Autodesk Inventor part; units mm, degrees
ref_plane "YZ Plane" through (0, 0, 0) normal (1, 0, 0) x (0, 1, 0)
ref_plane "XZ Plane" through (0, 0, 0) normal (0, 1, 0) x (-1, 0, 0)
ref_plane "XY Plane" through (0, 0, 0) normal (0, 0, 1) x (1, 0, 0)
sketch "Sketch7" plane through (0, 0, 0) normal (0, 0, 1) x (1, 0, 0)
  line L0 (125, -75) -> (-125, -75)
  line L1 (-125, -75) -> (-125, 75)
  line L2 (-125, 75) -> (125, 75)
  line L3 (125, 75) -> (125, -75)
  line L4 (125, -75) -> (-125, 75) construction
  line L5 (-125, -75) -> (125, 75) construction
  point P0 (0, 0)
  dimension "d15" = 250
  dimension "d16" = 150
extrude "Box Outside" add sketch "Sketch7" along normal blind 60
sketch "Sketch8" plane through (0, 0, 60) normal (0, 0, 1) x (1, 0, 0)
  line L0 (-122, 72) -> (122, 72)
  line L1 (122, 72) -> (122, -72)
  line L2 (122, -72) -> (-122, -72)
  line L3 (-122, -72) -> (-122, 72)
  line L4 (125, 75) -> (-125, 75)
  line L5 (-125, 75) -> (-125, -75)
  line L6 (-125, -75) -> (125, -75)
  line L7 (125, -75) -> (125, 75)
  point P0 (0, 0)
  dimension "d19" = 3
  dimension "d20" = 3
  dimension "d21" = 3
  dimension "d22" = 3
extrude "Box Cut" cut sketch "Sketch8" against normal blind 55 contours L0 L1 L2 L3
sketch "Sketch9" plane through (-122, -72, 60) normal (0, 1, 0) x (1, 0, 0)
  line L0 (0, 0) -> (10, 0)
  line L1 (10, 0) -> (10, 25)
  line L2 (10, 25) -> (0, 25)
  line L3 (0, 25) -> (0, 0)
  point P0 (122, 60)
  dimension "d25" = 10
  dimension "d26" = 25
extrude "ScrewHole Box LB" add sketch "Sketch9" along normal blind 15
sketch "Sketch10" plane through (-122, -72, 5) normal (0, 1, 0) x (1, 0, 0)
  line L0 (244, -55) -> (244, 0)
  line L1 (244, -55) -> (234, -55)
  line L2 (234, -55) -> (234, -30)
  line L3 (234, -30) -> (244, -30)
  line L4 (244, -30) -> (244, -55)
  point P0 (122, 5)
  dimension "d29" = 10
  dimension "d30" = 25
extrude "ScrewHole Box RB" add sketch "Sketch10" along normal blind 15
sketch "Sketch11" plane through (-122, 72, 60) normal (0, -1, 0) x (1, 0, 0)
  line L0 (0, 0) -> (244, 0)
  line L1 (0, 0) -> (10, 0)
  line L2 (10, 0) -> (10, -25)
  line L3 (10, -25) -> (0, -25)
  line L4 (0, -25) -> (0, 0)
  point P0 (122, -60)
  dimension "d33" = 10
  dimension "d34" = 25
extrude "ScrewHole Box LU" add sketch "Sketch11" along normal blind 15
sketch "Sketch13" plane through (122, -72, 5) normal (-1, 0, 0) x (0, 0, 1)
  line L0 (55, 144) -> (0, 144)
  line L1 (55, 144) -> (30, 144)
  line L2 (30, 144) -> (30, 129)
  line L3 (30, 129) -> (55, 129)
  line L4 (55, 129) -> (55, 144)
  point P0 (-5, 72)
  dimension "d37" = 25
  dimension "d38" = 15
extrude "ScrewHole Box RU" add sketch "Sketch13" along normal blind 10
sketch "Sketch27" plane through (0, 0, 60) normal (0, 0, 1) x (1, 0, 0)
  line L0 (-112, -72) -> (-112, -57)
  line L1 (-125, 75) -> (-125, -75)
  line L2 (-112, -57) -> (-125, -57)
  line L3 (-125, -57) -> (-125, -75)
  line L4 (-125, -75) -> (-112, -75)
  line L5 (-112, -75) -> (-112, -57)
  line L6 (-112, -57) -> (-125, -75)
  line L7 (-112, -75) -> (-125, -57)
  circle A0 centre (-118.5, -66) radius 2.4
  point P0 (0, 0)
  dimension "d84" = 4.8
extrude "Outside ScrewHole LB" cut sketch "Sketch27" against normal blind 26 contours A0 L7 L6 | L6 L7 A0 | A0 L6 L7 | L7 L6 A0
sketch "Sketch29" plane through (0, 0, 60) normal (0, 0, 1) x (1, 0, 0)
  line L0 (-112, -72) -> (-112, -57)
  line L1 (-125, -75) -> (125, -75)
  line L2 (-112, -57) -> (-125, -57)
  line L3 (-125, -57) -> (-125, -75)
  line L4 (-125, -75) -> (-112, -75)
  line L5 (-112, -75) -> (-112, -57)
  line L6 (-112, -57) -> (-125, -75)
  circle A0 centre (-118.5, -66) radius 2.4
  point P0 (0, 0)
extrude "ScrewRibbon LB" add sketch "Sketch29" against normal blind 2 contours A0 L6 | L6 A0
sketch "Sketch30" plane through (0, 0, 60) normal (0, 0, 1) x (1, 0, 0)
  line L0 (-122, -57) -> (-112, -57)
  line L1 (-125, -75) -> (125, -75)
  line L2 (-112, -57) -> (-125, -57)
  line L3 (-125, -57) -> (-125, -75)
  line L4 (-125, -75) -> (-112, -75)
  line L5 (-112, -75) -> (-112, -57)
  line L6 (-112, -57) -> (-125, -75)
  circle A0 centre (-118.5, -66) radius 1.7
  point P0 (0, 0)
  dimension "d92" = 3.4
extrude "Inside ScrewHole LB" cut sketch "Sketch30" against normal blind 24 contours A0 L6 | L6 A0
sketch "Sketch31" plane through (0, 0, 60) normal (0, 0, 1) x (1, 0, 0)
  line L0 (-125, 75) -> (-125, -75)
  line L1 (-112, 57) -> (-122, 57)
  line L2 (-125, 75) -> (-112, 75)
  line L3 (-112, 75) -> (-112, 57)
  line L4 (-112, 57) -> (-125, 57)
  line L5 (-125, 57) -> (-125, 75)
  line L6 (-125, 75) -> (-112, 57)
  circle A0 centre (-118.5, 66) radius 2.4
  point P0 (0, 0)
  dimension "d95" = 4.8
extrude "Outside ScrewHole LU" cut sketch "Sketch31" against normal blind 24 contours A0 L6 | L6 A0
sketch "Sketch32" plane through (0, 0, 60) normal (0, 0, 1) x (1, 0, 0)
  line L0 (-122, 57) -> (-112, 57)
  line L1 (-125, 75) -> (-125, -75)
  line L2 (-112, 57) -> (-125, 57)
  line L3 (-125, 57) -> (-125, 75)
  line L4 (-125, 75) -> (-112, 75)
  line L5 (-112, 75) -> (-112, 57)
  line L6 (-112, 75) -> (-125, 57)
  circle A0 centre (-118.5, 66) radius 2.4
  point P0 (0, 0)
  dimension "d98" = 4.8
extrude "ScrewRibbon LU" add sketch "Sketch32" against normal blind 2 contours A0 L6 | L6 A0
sketch "Sketch33" plane through (0, 0, 60) normal (0, 0, 1) x (1, 0, 0)
  line L0 (125, 75) -> (-125, 75)
  line L1 (-112, 57) -> (-122, 57)
  line L2 (-125, 75) -> (-112, 75)
  line L3 (-112, 75) -> (-112, 57)
  line L4 (-112, 57) -> (-125, 57)
  line L5 (-125, 57) -> (-125, 75)
  line L6 (-125, 75) -> (-112, 57)
  circle A0 centre (-118.5, 66) radius 1.7
  point P0 (0, 0)
  dimension "d101" = 3.4
extrude "Inside ScrewHole LU" cut sketch "Sketch33" against normal blind 21.75 contours A0 L6 | L6 A0
sketch "Sketch34" plane through (0, 0, 60) normal (0, 0, 1) x (1, 0, 0)
  line L0 (112, 57) -> (112, 72)
  line L1 (125, 75) -> (-125, 75)
  line L2 (112, 57) -> (125, 57)
  line L3 (125, 57) -> (125, 75)
  line L4 (125, 75) -> (112, 75)
  line L5 (112, 75) -> (112, 57)
  line L6 (125, 75) -> (112, 57)
  circle A0 centre (118.5, 66) radius 2.4
  point P0 (0, 0)
  dimension "d104" = 4.8
extrude "Outside ScrewHole RU" cut sketch "Sketch34" against normal blind 37 contours A0 L6 | L6 A0
sketch "Sketch35" plane through (0, 0, 60) normal (0, 0, 1) x (1, 0, 0)
  line L0 (125, -75) -> (125, 75)
  line L1 (122, 57) -> (112, 57)
  line L2 (125, 75) -> (112, 75)
  line L3 (112, 75) -> (112, 57)
  line L4 (112, 57) -> (125, 57)
  line L5 (125, 57) -> (125, 75)
  line L6 (125, 75) -> (-125, 75)
  line L7 (125, 75) -> (112, 57)
  circle A0 centre (118.5, 66) radius 2.4
  point P0 (0, 0)
  dimension "d107" = 4.8
extrude "ScrewRibbon RU" add sketch "Sketch35" against normal blind 2 contours A0 L7 | L7 A0
sketch "Sketch36" plane through (0, 0, 60) normal (0, 0, 1) x (1, 0, 0)
  line L0 (122, 57) -> (112, 57)
  line L1 (125, -75) -> (125, 75)
  line L2 (112, 57) -> (125, 57)
  line L3 (125, 57) -> (125, 75)
  line L4 (125, 75) -> (112, 75)
  line L5 (112, 75) -> (112, 57)
  line L6 (112, 57) -> (125, 75)
  circle A0 centre (118.5, 66) radius 2.4
  circle A1 centre (118.5, 66) radius 1.7
  point P0 (0, 0)
  dimension "d110" = 3.4
extrude "Inside ScrewHole RU" cut sketch "Sketch36" against normal blind 20 contours A1 L6 | L6 A1
sketch "Sketch37" plane through (0, 0, 60) normal (0, 0, 1) x (1, 0, 0)
  line L0 (125, -75) -> (125, 75)
  line L1 (112, -72) -> (112, -57)
  line L2 (125, -75) -> (112, -75)
  line L3 (112, -75) -> (112, -57)
  line L4 (112, -57) -> (125, -57)
  line L5 (125, -57) -> (125, -75)
  line L6 (112, -75) -> (125, -57)
  circle A0 centre (118.5, -66) radius 2.4
  point P0 (0, 0)
  dimension "d113" = 4.8
extrude "Outside ScrewHole RB" cut sketch "Sketch37" against normal blind 27.5 contours A0 L6 | L6 A0
sketch "Sketch38" plane through (0, 0, 60) normal (0, 0, 1) x (1, 0, 0)
  line L0 (122, -57) -> (112, -57)
  line L1 (125, -75) -> (125, 75)
  line L2 (112, -57) -> (125, -57)
  line L3 (125, -57) -> (125, -75)
  line L4 (125, -75) -> (112, -75)
  line L5 (112, -75) -> (112, -57)
  line L6 (125, -57) -> (112, -75)
  circle A0 centre (118.5, -66) radius 2.4
  point P0 (0, 0)
  dimension "d116" = 4.8
extrude "ScrewRibbon RB" add sketch "Sketch38" against normal blind 2 contours A0 L6 | L6 A0
sketch "Sketch39" plane through (0, 0, 60) normal (0, 0, 1) x (1, 0, 0)
  line L0 (112, -72) -> (112, -57)
  line L1 (125, -75) -> (125, 75)
  line L2 (112, -57) -> (125, -57)
  line L3 (125, -57) -> (125, -75)
  line L4 (125, -75) -> (112, -75)
  line L5 (112, -75) -> (112, -57)
  line L6 (112, -75) -> (125, -57)
  circle A0 centre (118.5, -66) radius 2.4
  circle A1 centre (118.5, -66) radius 1.7
  point P0 (0, 0)
  dimension "d119" = 3.4
extrude "Inside ScrewHole RB" cut sketch "Sketch39" against normal blind 20 contours A1 L6 | L6 A1
sketch "Sketch42" plane through (-122, -72, 5) normal (0, 1, 0) x (1, 0, 0)
  line L0 (244, 0) -> (0, 0)
  line L1 (12.5963, 0) -> (43.5963, 0)
  line L2 (43.5963, 0) -> (43.5963, -55)
  line L3 (43.5963, -55) -> (12.5963, -55)
  line L4 (12.5963, -55) -> (12.5963, 0)
  point P0 (122, 5)
  point P1 (43.5963, 0)
  dimension "d134" = 31
  dimension "d135" = 55
extrude "ESPHolder" add sketch "Sketch42" along normal blind 5
sketch "Sketch43" plane through (0, 0, 5) normal (0, 0, 1) x (1, 0, 0)
  line L0 (-109.4037, -67) -> (-78.4037, -67)
  line L1 (-99.1037, -67) -> (-88.7037, -67)
  line L2 (-88.7037, -67) -> (-88.7037, -62.5)
  line L3 (-88.7037, -62.5) -> (-99.1037, -62.5)
  line L4 (-99.1037, -62.5) -> (-99.1037, -67)
  line L5 (-78.4037, -67) -> (-109.4037, -67)
  line L6 (-109.4037, -67) -> (-109.4037, -51.7804)
  line L7 (-109.4037, -51.7804) -> (-78.4037, -51.7804)
  line L8 (-78.4037, -51.7804) -> (-78.4037, -67)
  point P0 (0, 0)
  dimension "d138" = 10.3
  dimension "d139" = 10.3
  dimension "d140" = 4.5
extrude "PortHole" cut sketch "Sketch43" against normal through all contours L4 L3 L2 L0
sketch "Sketch44" plane through (0, 0, 0) normal (0, 0, -1) x (-1, 0, 0)
  line L0 (84.7037, -58.5) -> (103.1037, -58.5)
  line L1 (103.1037, -58.5) -> (103.1037, -71)
  line L2 (103.1037, -71) -> (84.7037, -71)
  line L3 (84.7037, -71) -> (84.7037, -58.5)
  line L4 (88.7037, -62.5) -> (99.1037, -62.5)
  line L5 (99.1037, -67) -> (88.7037, -67)
  line L6 (99.1037, -62.5) -> (99.1037, -67)
  line L7 (88.7037, -67) -> (88.7037, -62.5)
  point P0 (0, 0)
  dimension "d143" = 4
  dimension "d144" = 4
  dimension "d145" = 4
  dimension "d146" = 4
extrude "Extrusion29" cut sketch "Sketch44" against normal blind 4
chamfer "Chamfer1" distance 15 angle 45 1 edges at (-117, -57, 35)
chamfer "Chamfer2" distance 15 angle 45 1 edges at (-117, 57, 35)
chamfer "Chamfer3" distance 15 angle 45 1 edges at (117, 57, 35)
chamfer "Chamfer4" distance 15 angle 45 1 edges at (117, -57, 35)
properties part number "Box2"
Design review of the part built by this model. Coordinates are the model's own, in mm. A direction names the side the tool comes from. Coordinates: 2 decimals unless noted, no trailing zeros. Order: outer loops, then holes, each group sorted by start corner. A loop starts at its lowest first (then second) coordinate and runs counter-clockwise, first axis right, second up. Notation, with made-up numbers: (30.5, 69.5) -> (80.5, 69.5) arc R22 cw to (80.5, 107.5) -> close; hole circle Ø3 at (82.25, 11). An arc over 180 degrees is marked (long way). Use one line per item in the form item = value. Start each with the question number.
(1) Add section C-C on x = 41.5. State the section outline as (y, z) points.
(2) Insertion check: pin 1 (2.5 mm diameter, centred on x = -118.5, y = 66, fed in from +Z); pin 2 (12 mm diameter, centred on x = -37, y = -10.5, fed in from -Z). Each pin has a flat end and moves straight along its axis. Give the tip position at first contact, or say it passes through.
(3) Add section A-A on z = 22.5. State the section outline as (x, y) points, plus the area to 3 significant figures.
(4) For faces 4 (the flat face through (-112, 66, 50)), 5 (the flat face through (-2, 1, 0)), 6 (the flat face through (-114, -72, 27)), list the 3-axis set-ups (+Z, -Z, +X, -X, +Y, -Y) from which the entire face can be reached by the end or side of a thin tool; tool diameter is ignored.
(5) Add section B-B on y = -24. State the section outline as (x, z) points, plus the area to 3 significant figures.
(6) The part is to be moulded in two halves that separate along X. For faces 1 (the flat face through (2, -75, 30)), 2 (the flat face through (-112, -66, 50)), 3 (the flat face through (125, 1, 30)), say which applies: +X half, -X half, draft (parallel to the pull), parting line (faces both ways), or undercut.
(7) For probe 1 along Y at (x, z) = (-118.5, 58.7); probe 2 along X at (y, z) = (-66, 46); probe 3 along Y at (x, z) = (118.5, 52.75), list the stretches that pass through material, from the lowest coordinate up.
Answer block:
q1.outline = (-75, 0) -> (75, 0) -> (75, 60) -> (72, 60) -> (72, 5) -> (-72, 5) -> (-72, 60) -> (-75, 60) -> close
q2.pin_1 = 5
q2.pin_2 = 0
q3.outline = (-125, -75) -> (125, -75) -> (125, 75) -> (-125, 75) -> close; hole (-122, -72) -> (-109.4, -72) -> (-109.4, -67) -> (-78.4, -67) -> (-78.4, -72) -> (122, -72) -> (122, 72) -> (-122, 72) -> close
q3.area = 2,520 mm²
q4.face_4 = +Z
q4.face_5 = -Z, +X, -X, +Y, -Y
q4.face_6 = none
q5.outline = (-125, 0) -> (125, 0) -> (125, 60) -> (122, 60) -> (122, 5) -> (-122, 5) -> (-122, 60) -> (-125, 60) -> close
q5.area = 1,580 mm²
q6.face_1 = draft
q6.face_2 = undercut
q6.face_3 = +X half
q7.probe_1 = -75 to -67.7, -64.3 to -57, 57 to 64.3, 67.7 to 75
q7.probe_2 = -125 to -120.9, -116.1 to -112, 112 to 116.1, 120.9 to 125
q7.probe_3 = -75 to -68.4, -63.6 to -57, 57 to 63.6, 68.4 to 75
